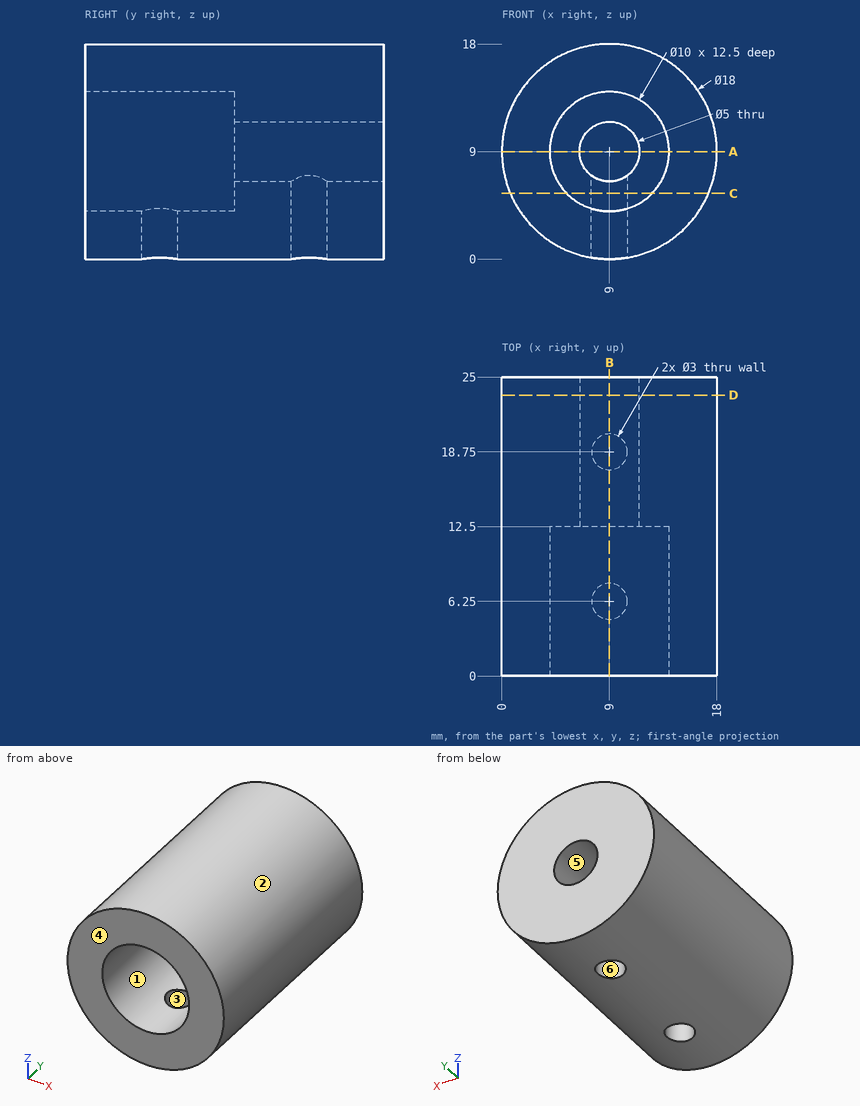
Could you check a few things on this drawing? It's one solid part, dimensions in mm from its lowest x, y, z. A direction names the side the tool comes from. Round coordinates to 2 decimals unless told otherwise and drop trailing zeros. Loops run counter-clockwise (first coordinate to the right, second up) from the corner with the lowest first, then second, coordinate; pieces in that order, holes last. Notation, with made-up numbers: (66, 21) -> (80, 21) arc R16 cw to (80, 28) -> close; hole circle Ø8 at (-14.5, -39.75). An arc over 180 degrees is marked (long way). Write each question's results on one line, items separated by ' | '.
(1) For the marked faces 1, 2 and 3, which set-ups out of +Z, -Z, +X, -X, +Y, -Y let a thin tool reach every point of the face, with its end or its side?
Worked answers:
face 1: -Y | face 2: +Y, -Y | face 3: -Z
(2) We'd pull the mould along Y, two halves only. Please class the marked faces 4, 5 and 6: released by +Y, released by -Y, zero draft, split by the parting line, or undercut.
Worked answers:
face 4: released by -Y | face 5: zero draft | face 6: undercut
(3) For P1, Ø2, axis at y = 15.5, z = 3.5, coming from the +X side; P2, Ø3, axis at x = 9, z = 9, coming from the -Y side; P3, Ø5, axis at x = 8.5, z = 10.5, coming from the -Y side; P4, Ø4, axis at y = 10.5, z = 6, coming from the +X side, each with a flat end and sliding along its axis, tell me the tip position at first contact or that it passes through.
Worked answers:
P1: x = 16.79 | P2: through | P3: y = 12.5 | P4: x = 17.94
(4) If we section it at B-B, the plane x = 9: List the corners of the cut face in (y, z) for me, then the cut area to 3 significant figures.
Worked answers:
outline: (0, 0) -> (4.75, 0) -> (4.75, 4) -> (0, 4) -> close; (0, 14) -> (12.5, 14) -> (12.5, 11.5) -> (25, 11.5) -> (25, 18) -> (0, 18) -> close; (7.75, 0) -> (17.25, 0) -> (17.25, 6.5) -> (12.5, 6.5) -> (12.5, 4) -> (7.75, 4) -> close; (20.25, 0) -> (25, 0) -> (25, 6.5) -> (20.25, 6.5) -> close | area: 231 mm2
(5) If we section it at A-A, the plane z = 9: List the corners of the cut face in (x, y) for me.
Worked answers:
outline: (0, 0) -> (4, 0) -> (4, 12.5) -> (6.5, 12.5) -> (6.5, 25) -> (0, 25) -> close; (11.5, 12.5) -> (14, 12.5) -> (14, 0) -> (18, 0) -> (18, 25) -> (11.5, 25) -> close
(6) If I drill on L1, parallel to Y at x = 9, z = 3; L2, parallel to Z at x = 9, y = 15.5; L3, parallel to Z at x = 9, y = 4.5, over which ranges is the centre line in solid material (lowest first)?
Worked answers:
L1: 0 to 4.75, 7.75 to 17.25, 20.25 to 25 | L2: 0 to 6.5, 11.5 to 18 | L3: 0 to 4, 14 to 18
(7) If we section it at D-D, the plane y = 23.5: List the corners of the cut face in (x, z) for me, then the cut area to 3 significant figures.
Worked answers:
outline: circle Ø18 at (9, 9); hole circle Ø5 at (9, 9) | area: 235 mm2
(8) If we section it at C-C, the plane z = 5.5: List the corners of the cut face in (x, y) for me, then the cut area to 3 significant figures.
Worked answers:
outline: (0.71, 0) -> (5.43, 0) -> (5.43, 12.5) -> (12.57, 12.5) -> (12.57, 0) -> (17.29, 0) -> (17.29, 25) -> (0.71, 25) -> close; hole circle Ø3 at (9, 18.75) | area: 318 mm2
